Study the drawing (mm; zero at the part's minimum x, y, z) and answer. Coordinates: 2 decimals unless noted, no trailing zeros. Write each loop counter-clockwise with the first axis right and the second up, starting at its lowest first coordinate (ties: lowest second). Pieces come first, ordered by that corner, then holes. Notation, with made-up numbers: (26, 73) -> (40, 73) arc R27 ccw to (40, 107) -> close; hole circle Ø2 at (70, 89.25). An arc over 180 degrees is marked (long way). Write each question's results on one line, items separated by ' | '. Start each with the question number.
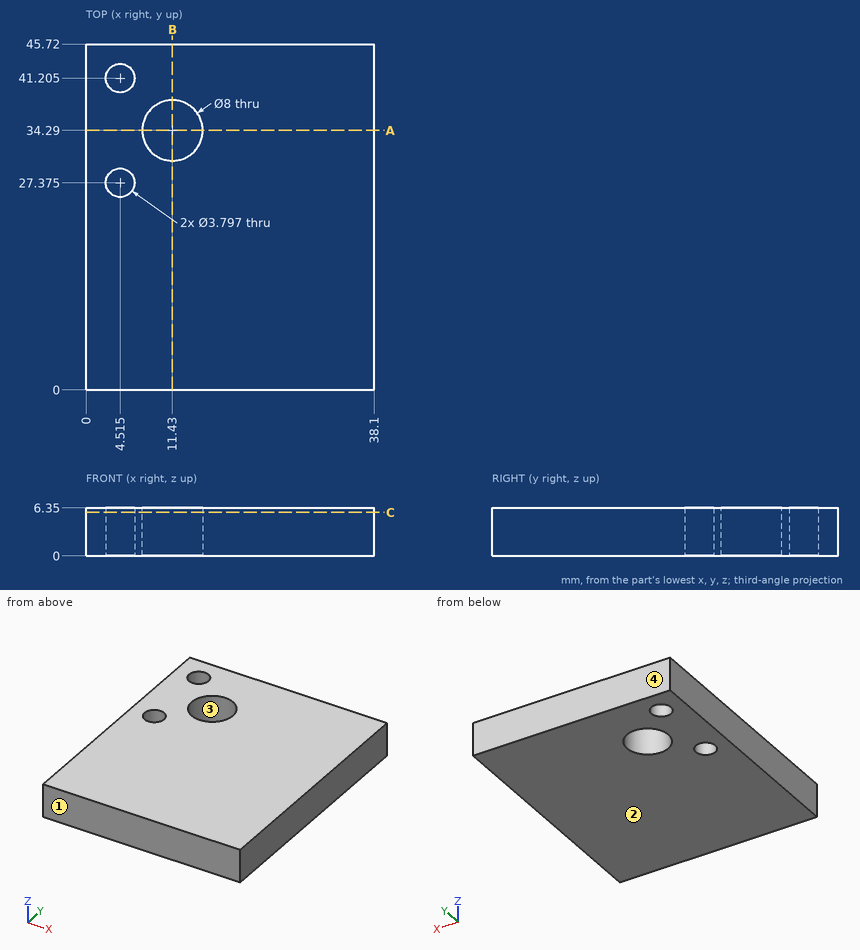
1. Determine the mould class of the marked faces 1, 2, 3 and 4 for opening direction Y: pulls with the +Y half, pulls with the -Y half, needs draft (parallel to the pull), parting line crosses it, or undercut.
2. Given pin 1 Ø5 at (x, y) = (11.43, 34.29) entering from +Z, flat-ended and moving along its own axis, determine where the tip first touches the part or whether it passes through.
3. Find the intervals of material crossed by L1, parallel to X at y = 28, z = 2; L2, parallel to Y at x = 12.5, z = 2 (1 decimal); L3, parallel to X at y = 29, z = 4.25 (1 decimal), in increasing order.
4. Find section B-B on x = 11.43. Give the vertices of the cut face in (y, z).
5. Find section C-C on z = 5.75. Give the vertices of the cut face in (x, y) (1 decimal), and give its area (3 significant figures).
6. Find section A-A on y = 34.29. Give the vertices of the cut face in (x, z), and give its area (3 significant figures).
Ans:
1) face 1: pulls with the -Y half | face 2: needs draft | face 3: undercut | face 4: pulls with the +Y half
2) pin 1: passes through
3) L1: x = 0 to 2.72, 6.31 to 38.1 | L2: y = 0 to 30.4, 38.1 to 45.7 | L3: x = 0 to 3.5, 5.5 to 38.1
4) outline: (0, 0) -> (30.29, 0) -> (30.29, 6.35) -> (0, 6.35) -> close; (38.29, 0) -> (45.72, 0) -> (45.72, 6.35) -> (38.29, 6.35) -> close
5) outline: (0, 0) -> (38.1, 0) -> (38.1, 45.7) -> (0, 45.7) -> close; hole circle Ø3.8 at (4.5, 27.4); hole circle Ø3.8 at (4.5, 41.2); hole circle Ø8 at (11.4, 34.3) | area: 1,670 mm²
6) outline: (0, 0) -> (7.43, 0) -> (7.43, 6.35) -> (0, 6.35) -> close; (15.43, 0) -> (38.1, 0) -> (38.1, 6.35) -> (15.43, 6.35) -> close | area: 191 mm²
